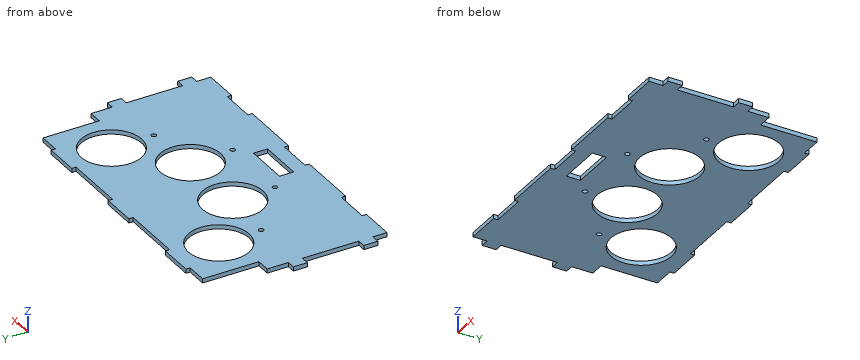
```python
from build123d import *

# Parameters (mm, degrees)
SKETCH_1_R      = 43
SKETCH_1_R_2    = 3.5
SKETCH_1_W      = 63
SKETCH_1_H      = 20
EXTRUDE_2_DEPTH = 6


with BuildPart() as part:
    # Эскиз1 → Бобышка-Вытянуть2 (new body)
    with BuildSketch(Plane.XY):
        Polygon((450, 20), (450, 40), (438, 40), (438, 120), (450, 120), (450, 140), (438, 140), (438, 170), (418, 170), (418, 250), (388, 250), (388, 256), (338, 256), (338, 250), (250, 250), (250, 256), (200, 256), (200, 250), (112, 250), (112, 256), (62, 256), (62, 250), (32, 250), (32, 170), (12, 170), (12, 140), (0, 140), (0, 120), (12, 120), (12, 40), (0, 40), (0, 20), (12, 20), (12, 0), (62, 0), (62, 6), (112, 6), (112, 0), (200, 0), (200, 6), (250, 6), (250, 0), (338, 0), (338, 6), (388, 6), (388, 0), (438, 0), (438, 20), align=None)
        with Locations((95.096189432, 190)):
            Circle(SKETCH_1_R, mode=Mode.SUBTRACT)
        with Locations((173.696978501, 124.046106882)):
            Circle(SKETCH_1_R, mode=Mode.SUBTRACT)
        with Locations((276.303021499, 124.046106882)):
            Circle(SKETCH_1_R, mode=Mode.SUBTRACT)
        with Locations((354.903810568, 190)):
            Circle(SKETCH_1_R, mode=Mode.SUBTRACT)
        with Locations((95.096189432, 130)):
            Circle(SKETCH_1_R_2, mode=Mode.SUBTRACT)
        with Locations((173.696978501, 64.046106882)):
            Circle(SKETCH_1_R_2, mode=Mode.SUBTRACT)
        with Locations((276.303021499, 64.046106882)):
            Circle(SKETCH_1_R_2, mode=Mode.SUBTRACT)
        with Locations((354.903810568, 130)):
            Circle(SKETCH_1_R_2, mode=Mode.SUBTRACT)
        with Locations((225, 36)):
            Rectangle(SKETCH_1_W, SKETCH_1_H, mode=Mode.SUBTRACT)
    extrude(amount=EXTRUDE_2_DEPTH)


solid = part.part
```
Verification items for the finished model (mm, model axes). Round coordinates to 2 decimals unless told otherwise and drop trailing zeros. Loops run counter-clockwise (first coordinate to the right, second up) from the corner with the lowest first, then second, coordinate; pieces in that order, holes last. Notation, with made-up numbers: (52.5, 86) -> (62.5, 86) arc R20 cw to (62.5, 97) -> close; hole circle Ø4 at (-8.75, 42). An arc over 180 degrees is marked (long way). Answer as a JSON object with one key per item and string values.
Q1. Scan lines: line 1 (X direction, y = 31.5, z = 3.25); line 2 (X direction, y = 130, z = 4.5); line 3 (X direction, y = 94, z = 2.9). Record each from-to range of solid material in increasing order. Write a range as from..to.
Data:
{"line 1": "x = 0..193.5, 256.5..450", "line 2": "x = 0..91.6, 98.6..131.11, 216.28..233.72, 318.89..351.4, 358.4..450", "line 3": "x = 12..142.94, 204.46..245.54, 307.06..438"}
Q2. Section check A-A (y = 190). Record the boundary of the cut face in (x, z).
Data:
{"outline": "(32, 0) -> (52.1, 0) -> (52.1, 6) -> (32, 6) -> close; (138.1, 0) -> (311.9, 0) -> (311.9, 6) -> (138.1, 6) -> close; (397.9, 0) -> (418, 0) -> (418, 6) -> (397.9, 6) -> close"}
Q3. Section check D-D (y = 95.5). Record the boundary of the cut face in (x, z), then the cut area to 3 significant figures.
Data:
{"outline": "(12, 0) -> (141.54, 0) -> (141.54, 6) -> (12, 6) -> close; (205.85, 0) -> (244.15, 0) -> (244.15, 6) -> (205.85, 6) -> close; (308.46, 0) -> (438, 0) -> (438, 6) -> (308.46, 6) -> close", "area": "1,780 mm2"}
Q4. Go/stop test with flat-tipped pins: P1, Ø1.8, axis at x = 425.5, z = 4, coming from the +Y side; P2, Ø3, axis at x = 4.5, z = 2.5, coming from the -Y side; P3, Ø1.8, axis at y = 85, z = 2.5, coming from the +X side; P4, Ø9, axis at x = 95.1, y = 130, coming from the +Z side. Record where each tip stops, or that it passes through.
Data:
{"P1": "stops at y = 170", "P2": "stops at y = 20", "P3": "stops at x = 438", "P4": "stops at z = 6"}
Q5. Section check B-B (x = 82). Record the boundary of the cut face in (y, z).
Data:
{"outline": "(6, 0) -> (149.04, 0) -> (149.04, 6) -> (6, 6) -> close; (230.96, 0) -> (256, 0) -> (256, 6) -> (230.96, 6) -> close"}
Q6. Section check C-C (y = 160). Record the boundary of the cut face in (x, z), then the cut area to 3 significant figures.
Data:
{"outline": "(12, 0) -> (64.29, 0) -> (64.29, 6) -> (12, 6) -> close; (125.9, 0) -> (150.11, 0) -> (150.11, 6) -> (125.9, 6) -> close; (197.28, 0) -> (252.72, 0) -> (252.72, 6) -> (197.28, 6) -> close; (299.89, 0) -> (324.1, 0) -> (324.1, 6) -> (299.89, 6) -> close; (385.71, 0) -> (438, 0) -> (438, 6) -> (385.71, 6) -> close", "area": "1,250 mm2"}
